```python
from build123d import *

# Parameters (mm, degrees)
SKIZZE1_R                       = 5
AUFSATZ_LINEAR_AUSTRAGEN1_DEPTH = 53
SKIZZE2_R                       = 3
SCHNITT_LINEAR_AUSTRAGEN1_DEPTH = 47
FASE1_SIZE                      = 1


with BuildPart() as part:
    # Skizze1 → Aufsatz-Linear austragen1 (new body)
    with BuildSketch(Plane.XY):
        Circle(SKIZZE1_R)
    extrude(amount=AUFSATZ_LINEAR_AUSTRAGEN1_DEPTH)

    # Skizze2 → Schnitt-Linear austragen1 (cut)
    with BuildSketch(Plane(origin=(0, 5, 0), x_dir=(1, 0, 0), z_dir=(0, 1, 0))):
        with Locations(Location((0, -5, 0), (0, 0, 270))):
            Circle(SKIZZE2_R)
        with Locations(Location((0, -48, 0), (0, 0, 270))):
            Circle(SKIZZE2_R)
    extrude(amount=-SCHNITT_LINEAR_AUSTRAGEN1_DEPTH, mode=Mode.SUBTRACT)

    # Fase1
    fase1_edges = [part.edges().sort_by_distance(p)[0] for p in [
        (-5, 0, 0),
        (-5, 0, 53),
    ]]
    chamfer(fase1_edges, length=FASE1_SIZE)


solid = part.part
```
Read the model definition and answer for the solid it produces. Units are mm, in the model's axes. Coordinates: 2 decimals unless noted, no trailing zeros. Order: outer loops, then holes, each group sorted by start corner. A loop starts at its lowest first (then second) coordinate and runs counter-clockwise, first axis right, second up. Notation, with made-up numbers: (30, 2.5) - (79, 2.5) arc R13 cw to (79, 26.5) - close; hole circle Ø11 at (9.25, 80.5). An arc over 180 degrees is marked (long way). Answer as a JSON object with one key per item and string values. Group by question number.
Item 1: Consider probe 1 along Z at (x, y) = (0, -1.25); probe 2 along X at (y, z) = (0.25, 48); probe 3 along Z at (x, y) = (1.25, -0.75). Determine where each line is inside the solid, lowest interval first. Write a range as from..to.
Item 2: A flat-ended cylindrical pin translates along its axis: P1, Ø1.5, axis at y = -2, z = 14, coming from the -X side. Find the tip coordinate at first contact, or state that the pin passes through.
Item 3: Section B-B (y = 0) is taken. Give the vertices of the cut face in (x, z).
Item 4: Section A-A (x = 0) is taken. Give the vertices of the cut face in (y, z).
Item 5: The mould has two halves that part along Z. Classify faces 1 (the face through (0, 0, 45)), 2 (the face through (0, 0, 0)), 3 (the face through (0, 0, 53)), 4 (the face through (0, 0, 2)): +Z half, -Z half, draft (parallel to the pull), parting line (faces both ways), or undercut.
Item 6: Section D-D (y = -2.75) is taken. State how many separate pieces and enclosed holes the cut face has, plus the area to 3 significant figures.
Item 7: Section C-C (z = 5) is taken. Give the vertices of the cut face in (x, y), plus the area to 3 significant figures.
Results are:
{
 "1": {"probe 1": "z = 0..2, 8..45, 51..53", "probe 2": "x = -4.99..-3, 3..4.99", "probe 3": "z = 0..2.27, 7.73..45.27, 50.73..53"},
 "2": {"P1": "stops at x = -4.84"},
 "3": {"outline": "(-5, 1) - (-4, 0) - (4, 0) - (5, 1) - (5, 52) - (4, 53) - (-4, 53) - (-5, 52) - close; hole circle Ø6 at (0, 5); hole circle Ø6 at (0, 48)"},
 "4": {"outline": "(-5, 1) - (-4, 0) - (4, 0) - (5, 1) - (5, 2) - (-5, 2) - close; (-5, 8) - (5, 8) - (5, 45) - (-5, 45) - close; (-5, 51) - (5, 51) - (5, 52) - (4, 53) - (-4, 53) - (-5, 52) - close"},
 "5": {"face 1": "undercut", "face 2": "-Z half", "face 3": "+Z half", "face 4": "undercut"},
 "6": {"separate pieces": "1", "enclosed holes": "2", "area": "384 mm^2"},
 "7": {"outline": "(-3, -4) - (-3, 4) arc R5 ccw to start; (3, -4) arc R5 ccw to (3, 4) - close", "area": "22.4 mm^2"}
}
